```python
from build123d import *

# Parameters (mm, degrees)
F0_R     = 12.7
F1_DEPTH = 279.4
F3_DEPTH = 2.54


with BuildPart() as f1:
    # F0 (on Right) → F1 (new body)
    with BuildSketch(Plane.YZ):
        Circle(F0_R)
    extrude(amount=F1_DEPTH)

    # F2 (on face) → F3 (cut)
    with BuildSketch(Plane.YZ.offset(279.4)):
        with BuildLine():
            ThreePointArc((5.696123, -2.806543), (6.184371, -1.440854), (6.35, 0))
            ThreePointArc((6.35, 0), (6.184371, 1.440854), (5.696123, 2.806543))
            ThreePointArc((5.696123, 2.806543), (4.755533, 4.208017), (3.478958, 5.312189))
            ThreePointArc((3.478958, 5.312189), (0, 6.35), (-3.478958, 5.312189))
            ThreePointArc((-3.478958, 5.312189), (-4.755533, 4.208017), (-5.696123, 2.806543))
            ThreePointArc((-5.696123, 2.806543), (-6.35, 0), (-5.696123, -2.806543))
            ThreePointArc((-5.696123, -2.806543), (-4.755533, -4.208017), (-3.478958, -5.312189))
            ThreePointArc((-3.478958, -5.312189), (0, -6.35), (3.478958, -5.312189))
            ThreePointArc((3.478958, -5.312189), (4.755533, -4.208017), (5.696123, -2.806543))
        make_face()
        with BuildLine():
            ThreePointArc((5.696123, 2.806543), (6.184371, 1.440854), (6.35, 0))
            ThreePointArc((6.35, 0), (6.184371, -1.440854), (5.696123, -2.806543))
            Line((5.696123, -2.806543), (28.013255, -2.806543))
            Line((28.013255, -2.806543), (28.013255, 0))
            Line((28.013255, 0), (28.013255, 2.806543))
            Line((28.013255, 2.806543), (5.696123, 2.806543))
        make_face()
        with BuildLine():
            ThreePointArc((-3.478958, 5.312189), (0, 6.35), (3.478958, 5.312189))
            Line((3.478958, 5.312189), (3.478958, 26.45749))
            Line((3.478958, 26.45749), (0, 26.45749))
            Line((0, 26.45749), (-3.478958, 26.45749))
            Line((-3.478958, 26.45749), (-3.478958, 5.312189))
        make_face()
        with BuildLine():
            Line((3.478958, -31.876493), (3.478958, -5.312189))
            ThreePointArc((3.478958, -5.312189), (0, -6.35), (-3.478958, -5.312189))
            Line((-3.478958, -5.312189), (-3.478958, -31.876493))
            Line((-3.478958, -31.876493), (0, -31.876493))
            Line((0, -31.876493), (3.478958, -31.876493))
        make_face()
        with BuildLine():
            ThreePointArc((-5.696123, -2.806543), (-6.35, 0), (-5.696123, 2.806543))
            Line((-5.696123, 2.806543), (-29.619023, 2.806543))
            Line((-29.619023, 2.806543), (-29.619023, 0))
            Line((-29.619023, 0), (-29.619023, -2.806543))
            Line((-29.619023, -2.806543), (-5.696123, -2.806543))
        make_face()
    extrude(amount=-F3_DEPTH, mode=Mode.SUBTRACT)


solid = f1.part
```
The listing builds one solid part. Answer for the finished solid, in the listing's coordinates (mm). Coordinates: 2 decimals unless noted, no trailing zeros. Write each loop counter-clockwise with the first axis right and the second up, starting at its lowest first coordinate (ties: lowest second). Pieces come first, ordered by that corner, then holes.
Q1. The mould has two halves that part along Y. Classify faces 1 (the flat face through (0, 0, 0)), 2 (the flat face through (276.86, 0, 0)), 3 (the cylindrical face through (137.74, -2.75, -12.4)): released by +Y, released by -Y, zero draft, split by the parting line, or undercut.
Returned:
face 1: zero draft
face 2: undercut
face 3: split by the parting line
Q2. Find the intervals of material crossed by line 1 along X through (y, z) = (-7.25, 2); line 2 along Z through (x, y) = (190, -1); line 3 along Y through (x, z) = (162.5, -3), in increasing order.
Returned:
line 1: x = 0 to 276.86
line 2: z = -12.66 to 12.66
line 3: y = -12.34 to 12.34
Q3. Section B-B, the plane y = -8.5 is taken. Write down the section's boundary in (x, z), then the cut area to 3 significant figures.
Returned:
outline: (0, -9.44) - (279.4, -9.44) - (279.4, -2.81) - (276.86, -2.81) - (276.86, 2.81) - (279.4, 2.81) - (279.4, 9.44) - (0, 9.44) - close
area: 5,260 mm2
Q4. Given P1, Ø3, axis at x = 142, y = -5, coming from the +Z side; P2, Ø0.8, axis at x = 278, y = -7.5, coming from the -Z side; P3, Ø3, axis at x = 278, y = -10.5, coming from the +Z side, each flat-ended and moving along its own axis, determine where each tip first touches the part or whether it passes through.
Returned:
P1: stops at z = 12.21
P2: stops at z = -10.53
P3: stops at z = 8.96
Q5. Section A-A, the plane x = 250 is taken. Write down the section's boundary in (y, z), then the cut area to 3 significant figures.
Returned:
outline: circle Ø25.4 at (0, 0)
area: 507 mm2
